The listing builds one solid part. Answer for the finished solid, in the listing's coordinates (mm). Face numbers are marked on the shaded views. A direction names the side the tool comes from. Coordinates: 2 decimals unless noted, no trailing zeros. Loops run counter-clockwise (first coordinate to the right, second up) from the corner with the lowest first, then second, coordinate; pieces in that order, holes last. Notation, with made-up numbers: M 65,-3.5 L 94,-3.5 A21 cw 94,32.5 Z; hole C -22.75,-33.5 d11. An arc over 180 degrees is marked long. Answer in a Markdown table with one row per item. Add a question column.
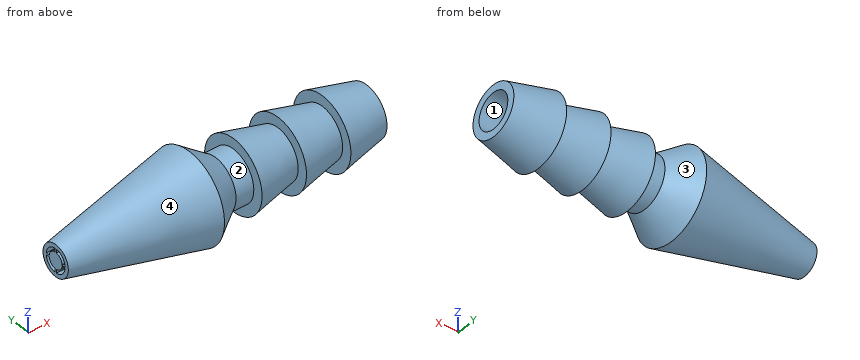
from build123d import *

# Parameters (mm, degrees)
SKETCH1_R           = 4
BOSS_EXTRUDE1_DEPTH = 5
BOSS_EXTRUDE1_TAPER = 13
SKETCH2_R           = 4
BOSS_EXTRUDE2_DEPTH = 5
BOSS_EXTRUDE2_TAPER = 13
SKETCH3_R           = 4
BOSS_EXTRUDE3_DEPTH = 5
BOSS_EXTRUDE3_TAPER = 13
SKETCH4_R           = 2.85
BOSS_EXTRUDE4_DEPTH = 2
SKETCH5_R           = 2.85
BOSS_EXTRUDE5_DEPTH = 3
BOSS_EXTRUDE5_DRAFT = -35
SKETCH6_R           = 4.950622615
BOSS_EXTRUDE6_DEPTH = 15
BOSS_EXTRUDE6_TAPER = 12
SKETCH9_R           = 2
CUT_EXTRUDE1_DEPTH  = 20
SKETCH14_R          = 2
CUT_EXTRUDE11_DEPTH = 10
CUT_EXTRUDE11_TAPER = 11.2
CUT_EXTRUDE13_DEPTH = 10


with BuildPart() as part:
    # Sketch1 → Boss-Extrude1 (new body)
    with BuildSketch(Plane(origin=(0, 0, 0), x_dir=(0, 0, -1), z_dir=(1, 0, 0))):
        Circle(SKETCH1_R)
    extrude(amount=BOSS_EXTRUDE1_DEPTH, taper=BOSS_EXTRUDE1_TAPER)

    # Sketch2 → Boss-Extrude2 (add)
    with BuildSketch(Plane(origin=(5, 0, 0), x_dir=(0, 0, -1), z_dir=(1, 0, 0))):
        Circle(SKETCH2_R)
    extrude(amount=BOSS_EXTRUDE2_DEPTH, taper=BOSS_EXTRUDE2_TAPER)

    # Sketch3 → Boss-Extrude3 (add)
    with BuildSketch(Plane(origin=(10, 0, 0), x_dir=(0, 0, -1), z_dir=(1, 0, 0))):
        Circle(SKETCH3_R)
    extrude(amount=BOSS_EXTRUDE3_DEPTH, taper=BOSS_EXTRUDE3_TAPER)

    # Sketch4 → Boss-Extrude4 (add)
    with BuildSketch(Plane.ZY):
        Circle(SKETCH4_R)
    extrude(amount=BOSS_EXTRUDE4_DEPTH)


with BuildPart() as boss_extrude5_tool:
    # Sketch5 → Boss-Extrude5 (with draft: the straight prism first)
    with BuildSketch(Plane.ZY.offset(2)):
        Circle(SKETCH5_R)
    extrude(amount=BOSS_EXTRUDE5_DEPTH)
    # Boss-Extrude5: the draft: its side faces are tilted about the plane it starts from
    boss_extrude5_sides = [boss_extrude5_tool.faces().sort_by_distance(p)[0] for p in [
        (-3.5, 0, -2.85),
    ]]
    draft(boss_extrude5_sides, Plane.ZY.offset(2), BOSS_EXTRUDE5_DRAFT)


with BuildPart() as part_1:
    add(part.part)

    # Boss-Extrude5: add boss_extrude5_tool
    add(boss_extrude5_tool.part)

    # Sketch6 → Boss-Extrude6 (add)
    with BuildSketch(Plane.ZY.offset(5)):
        Circle(SKETCH6_R)
    extrude(amount=BOSS_EXTRUDE6_DEPTH, taper=BOSS_EXTRUDE6_TAPER)

    # Sketch9 → Cut-Extrude1 (cut)
    with BuildSketch(Plane(origin=(15, 0, 0), x_dir=(0, 0, -1), z_dir=(1, 0, 0))):
        Circle(SKETCH9_R)
    extrude(amount=-CUT_EXTRUDE1_DEPTH, mode=Mode.SUBTRACT)

    # Sketch14 → Cut-Extrude11 (cut)
    with BuildSketch(Plane(origin=(-5, 0, 0), x_dir=(0, 0, -1), z_dir=(1, 0, 0))):
        Circle(SKETCH14_R)
    extrude(amount=-CUT_EXTRUDE11_DEPTH, taper=CUT_EXTRUDE11_TAPER, mode=Mode.SUBTRACT)

    # Sketch15 → Cut-Extrude13 (cut)
    with BuildSketch(Plane.ZY.offset(20)):
        with BuildLine():
            Line((-0.105022345, 0.89385139), (-0.105022345, 1.304678892))
            ThreePointArc((-0.105022345, 1.304678892), (-0.930174079, 0.920865292), (-1.305669179, 0.091895032))
            Line((-1.305669179, 0.091895032), (-0.89529621, 0.091895032))
            ThreePointArc((-0.89529621, 0.091895032), (-0.641048206, 0.631709741), (-0.105022345, 0.89385139))
        make_face()
        with BuildLine():
            ThreePointArc((1.305669179, 0.091895032), (0.932933814, 0.91806928), (0.112852256, 1.30402495))
            Line((0.112852256, 1.30402495), (0.112852256, 0.892896617))
            ThreePointArc((0.112852256, 0.892896617), (0.643810311, 0.628894493), (0.89529621, 0.091895032))
            Line((0.89529621, 0.091895032), (1.305669179, 0.091895032))
        make_face()
        with BuildLine():
            Line((-0.89529621, -0.091895032), (-1.305669179, -0.091895032))
            ThreePointArc((-1.305669179, -0.091895032), (-0.930174079, -0.920865292), (-0.105022345, -1.304678892))
            Line((-0.105022345, -1.304678892), (-0.105022345, -0.89385139))
            ThreePointArc((-0.105022345, -0.89385139), (-0.641048206, -0.631709741), (-0.89529621, -0.091895032))
        make_face()
        with BuildLine():
            ThreePointArc((0, -1.308899042), (0.892450386, -0.95747011), (1.305669179, -0.091895032))
            Line((1.305669179, -0.091895032), (0.89529621, -0.091895032))
            ThreePointArc((0.89529621, -0.091895032), (0.643810311, -0.628894493), (0.112852256, -0.892896617))
            ThreePointArc((0.112852256, -0.892896617), (0.056537797, -0.898222399), (0, -0.9))
            Line((0, -0.9), (0, -1.308899042))
        make_face()
    extrude(amount=-CUT_EXTRUDE13_DEPTH, mode=Mode.SUBTRACT)


solid = part_1.part
(1) A cutting plane is placed at B-B (x = 10.5). Give the vertices of the cut face in (y, z), plus the area to 3 significant figures.
(2) The mould has two halves that part along Z. Classify the marked faces 1 and 2: released by +Z, released by -Z, zero draft, split by the parting line, or undercut.
(3) A cutting plane is placed at A-A (x = -14). Give the vertices of the cut face in (y, z), plus the area to 3 significant figures.
(4) For the marked faces 3 and 4, determine the directions among +Z, -Z, +X, -X, +Y, -Y from which every point of the face is accessible in a straight line to the end or side of a thin tool.
(5) A cutting plane is placed at C-C (x = -5.5). Give the vertices of the cut face in (y, z).
(6) Straight lines are drawn through the part: line 1 (Z direction, x = 0.5, y = -1.25); line 2 (Y direction, x = 10.5, z = 0); line 3 (Y direction, x = -13, z = 0.75). For each, find the intervals that lie inside material, in ascending order.
(7) Each of these flat-tipped pins is pushed along its axis until it touches: pin 1 (5 mm diameter, centred on x = -5, z = 4, fed in from -Y); pin 2 (1.5 mm diameter, centred on x = -11, y = -1, fed in from +Z). Where does it stop, or does it pass through?
Solved:
| question | item | result |
|---|---|---|
| 1 | outline | C 0,0 d7.77; hole C 0,0 d4 |
| 1 | area | 34.8 mm² |
| 2 | face 1 | undercut |
| 2 | face 2 | split by the parting line |
| 3 | outline | C 0,0 d6.08; hole M -1.31,0 L -0.9,0 A0.9 cw -0.09,0.9 L -0.09,1.31 A1.31 ccw Z; hole M -1.3,-0.11 A1.31 ccw -0.09,-1.31 L -0.09,-0.9 A0.9 cw -0.89,-0.11 Z; hole C 0,0 d0.44; hole M 0.09,-1.31 A1.31 ccw 1.3,-0.11 L 0.89,-0.11 A0.9 cw 0.09,-0.9 Z; hole M 0.09,0.9 A0.9 cw 0.89,0.11 L 1.3,0.11 A1.31 ccw 0.09,1.31 Z |
| 3 | area | 26.3 mm² |
| 4 | face 3 | none |
| 4 | face 4 | -X |
| 5 | outline | C 0,0 d9.69; hole C 0,0 d3.8 |
| 6 | line 1 | z = -3.68 to -1.56, 1.56 to 3.68 |
| 6 | line 2 | y = -3.88 to -2, 2 to 3.88 |
| 6 | line 3 | y = -3.16 to -1.07, -0.5 to 0.5, 1.07 to 3.16 |
| 7 | pin 1 | stops at y = -4.72 |
| 7 | pin 2 | stops at z = 3.76 |
